Autodesk Inventor part; units mm, degrees
ref_plane "YZ Plane" through (0, 0, 0) normal (1, 0, 0) x (0, 1, 0)
ref_plane "XZ Plane" through (0, 0, 0) normal (0, 1, 0) x (-1, 0, 0)
ref_plane "XY Plane" through (0, 0, 0) normal (0, 0, 1) x (1, 0, 0)
sketch "Sketch1" plane through (0, 0, 0) normal (0, 0, 1) x (1, 0, 0)
  circle A0 centre (0, 0) radius 30
  dimension "d0" = 60
extrude "Extrusion1" add sketch "Sketch1" along normal blind 3
sketch "Sketch2" plane through (0, 0, 0) normal (0, 0, -1) x (-1, 0, 0)
  arc A0 (0, 12) -> (0, -18) centre (0, -3) ccw
  arc A1 (0, -12) -> (0, 18) centre (0, 3) ccw
  circle A2 centre (0, 0) radius 30
  line L0 (0, -18) -> (0, -12)
  line L1 (0, 12) -> (0, 18)
  dimension "d3" = 15
  dimension "d5" = 3
  dimension "d6" = 3
extrude "Extrusion2" add sketch "Sketch2" along normal blind 3 contours L1 A1 L0 A0
sketch "Sketch3" plane through (0, 0, 3) normal (0, 0, 1) x (1, 0, 0)
  point P0 (0, 0)
  point P1 (0, 0)
hole "Hole1" at (0, 0, 3) direction (0, 0, -1) diameter 1 end through all
equation "\"d0\" = rs_diametro"
equation "\"d1\" = rs_grosor"
equation "\"d3\" = 0.5 * rs_gancho_diametro"
equation "\"d7\" = rs_gancho_grosor"
equation "\"d9\" = ri_ancla_diametro"
properties part number "Rueda Superior"
Verification items for the finished model (mm, model axes). A direction names the side the tool comes from. Give positions to 0.01 mm unless a question says otherwise; leave off trailing zeros. Write each loop counter-clockwise with the first axis right and the second up, starting at its lowest first coordinate (ties: lowest second). Pieces come first, ordered by that corner, then holes. Notation, with made-up numbers: M 68.25,-14.5 L 74.25,-14.5 A17 cw 74.25,-10.5 Z; hole C 19.25,76 d5. An arc over 180 degrees is marked long. Put each result on its own line as item: value. Start each with the question number.
1. Section check A-A (z = 1.95). Record the cut outline in (x, y), and give its area (3 significant figures).
2. Set-up check for faces 4 (the face through (-29.97, -1.32, 1.48)), 5 (the face through (15, -3, -1)), 6 (the face through (0, -15, -1)): record each of +Z, -Z, +X, -X, +Y, -Y from which the full face is reachable in a straight line by a thin tool's end or side.
3. Go/stop test with flat-tipped pins: pin 1 Ø1.5 at (y, z) = (-16, -1) entering from -X; pin 2 Ø1.5 at (x, z) = (-2, 1) entering from +Y; pin 3 Ø3.5 at (y, z) = (16, -1) entering from +X. Record where each tip stops, or that it passes through.
4. Section check C-C (x = -1.5). Record the cut outline in (y, z), and give its area (3 significant figures).
5. Section check B-B (y = 4). Record the cut outline in (x, z), and give its area (3 significant figures).
6. Scan lines: line 1 along Y through (x, z) = (0, 1.1); line 2 along Z through (x, y) = (-3, -26.5); line 3 along X through (y, z) = (0, -0.65). Record each from-to range of solid material in increasing order. Write a range as [from, to].
7. Draft check along X on faces 1 (the face through (-3, 0, -3)), 2 (the face through (0, 15, -1)), 3 (the face through (-15, 3, -1)). Enter one of: +X half, -X half, draft (parallel to the pull), parting line (faces both ways), or undercut.
8. Section check D-D (z = -1.65). Record the cut outline in (x, y).
Answer list:
1. outline: C 0,0 d60; hole C 0,0 d1
1. area: 2,830 mm2
2. face 4: +Z, -Z
2. face 5: -Z, +X
2. face 6: -Z, -X, -Y
3. pin 1: x = 0
3. pin 2: y = 29.97
3. pin 3: x = 26.23
4. outline: M -29.96,0 L -11.92,0 L -11.92,-3 L 17.92,-3 L 17.92,0 L 29.96,0 L 29.96,3 L -29.96,3 Z
4. area: 269 mm2
5. outline: M -29.73,0 L -14.97,0 L -14.97,-3 L 13.27,-3 L 13.27,0 L 29.73,0 L 29.73,3 L -29.73,3 Z
5. area: 263 mm2
6. line 1: [-30, -0.5], [0.5, 30]
6. line 2: [0, 3]
6. line 3: [-14.7, -0.5], [0.5, 14.7]
7. face 1: draft
7. face 2: +X half
7. face 3: -X half
8. outline: M 0,-18 A15 ccw 0,12 L 0,18 A15 ccw 0,-12 Z; hole C 0,0 d1
